Geometry: final body of the model. Coordinates: model frame, mm. Face numbers are marked on the shaded views. A direction names the side the tool comes from. Give positions to 0.01 mm unless a question says otherwise; leave off trailing zeros. Write each loop counter-clockwise with the first axis right and the second up, starting at its lowest first coordinate (ties: lowest second). Pieces come first, ordered by that corner, then holes.
Solid Edge part; units mm, degrees
sketch "Sketch1" plane through (0, 0, 0) normal (0, 0, 1) x (1, 0, 0)
  circle A0 centre (0, 0) radius 12.165
extrude "Protrusion1" add sketch "Sketch1" along normal blind 11
sketch "Sketch2" plane through (0, 0, 11) normal (0, 0, 1) x (1, 0, 0)
  line L0 (0, -4.6188) -> (-4, -2.3094)
  line L1 (-4, -2.3094) -> (-4, 2.3094)
  line L2 (-4, 2.3094) -> (0, 4.6188)
  line L3 (0, 4.6188) -> (4, 2.3094)
  line L4 (4, 2.3094) -> (4, -2.3094)
  line L5 (4, -2.3094) -> (0, -4.6188)
extrude "Cutout1" cut sketch "Sketch2" against normal blind 5.5
sketch "Sketch3" plane through (0, 0, 0) normal (0, 0, -1) x (0, 1, 0)
  circle A0 centre (0, 0) radius 8
extrude "Protrusion2" add sketch "Sketch3" along normal blind 50
sketch "Sketch4" plane through (0, 0, -50) normal (0, 0, -1) x (0, 1, 0)
  circle A0 centre (0, 0) radius 6
extrude "Protrusion3" add sketch "Sketch4" along normal blind 18
chamfer "Chamfer1" distance 0.5 angle 45 1 edges at (0, -6, -68)
properties part number "131785"
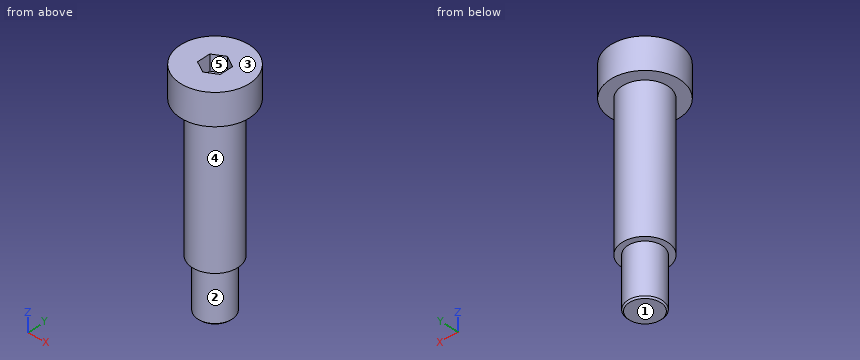
Item 1: Pull-direction query (X, two-part tool) for the marked faces 3, 4 and 5; classes: +X half, -X half, draft (parallel to the pull), parting line (faces both ways), or undercut.
Found:
face 3: draft
face 4: parting line
face 5: undercut
Item 2: Reachability of the marked faces 1 and 2 from +Z, -Z, +X, -X, +Y, -Y: full face, straight path, thin tool, end or side. Return the list, or none.
Found:
face 1: -Z, +X, -X, +Y, -Y
face 2: -Z
Item 3: Line query: L1, parallel to Z at x = -9.5, y = 4; L2, parallel to Z at x = -3.25, y = 6.5; L3, parallel to X at y = -1.75, z = -26. Output: solid intervals per line, ascending.
Found:
L1: z = 0 to 11
L2: z = -50 to 11
L3: x = -7.81 to 7.81
Item 4: Section D-D, the plane z = -57.5. Return the cut outline in (x, y).
Found:
outline: circle Ø12 at (0, 0)
Item 5: Section C-C, the plane x = -10. Return the cut outline in (y, z), plus the area to 3 significant figures.
Found:
outline: (-6.93, 0) - (6.93, 0) - (6.93, 11) - (-6.93, 11) - close
area: 152 mm2
Item 6: Pin query (flat end, axial travel): pin 1 Ø6 at (y, z) = (5.5, -12) entering from -X; pin 2 Ø4 at (x, y) = (6, -5) entering from -Z; pin 3 Ø4 at (x, y) = (1, -1.5) entering from +Z. Return the tip coordinate at first contact, or that it passes through.
Found:
pin 1: stops at x = -7.6
pin 2: stops at z = -67.69
pin 3: stops at z = 5.5
Item 7: Section A-A, the plane y = 0. Return the cut outline in (x, z) (3 decimals).
Found:
outline: (-12.165, 0) - (-8, 0) - (-8, -50) - (-6, -50) - (-6, -67.5) - (-5.5, -68) - (5.5, -68) - (6, -67.5) - (6, -50) - (8, -50) - (8, 0) - (12.165, 0) - (12.165, 11) - (4, 11) - (4, 5.5) - (-4, 5.5) - (-4, 11) - (-12.165, 11) - close
Item 8: Section B-B, the plane z = -32. Return the cut outline in (x, y).
Found:
outline: circle Ø16 at (0, 0)
